```python
from build123d import *

# Parameters (mm, degrees)
SKETCH1_W                  = 84.86693599
SKETCH1_H                  = 63.5
SKETCH1_R                  = 5.08
BOSS_EXTRUDE1_DEPTH        = 3.175
F_10_32_TAPPED_HOLE1_D     = 4.0386
F_10_32_TAPPED_HOLE1_DEPTH = 11.938
F_10_32_TAPPED_HOLE1_TIP   = 1.213317848
F_10_32_TAPPED_HOLE2_D     = 4.0386
F_10_32_TAPPED_HOLE2_DEPTH = 11.938
F_10_32_TAPPED_HOLE2_TIP   = 1.213317848
SKETCH10_W                 = 84.86693599
SKETCH10_H                 = 3.175
BOSS_EXTRUDE2_DEPTH        = 22.225
F_10_32_TAPPED_HOLE3_D     = 4.0386
F_10_32_TAPPED_HOLE3_DEPTH = 11.938
F_10_32_TAPPED_HOLE3_TIP   = 1.213317848
F_10_32_TAPPED_HOLE4_D     = 4.0386
F_10_32_TAPPED_HOLE4_DEPTH = 11.938
F_10_32_TAPPED_HOLE4_TIP   = 1.213317848


with BuildPart() as part:
    # Sketch1 → Boss-Extrude1 (new body)
    with BuildSketch(Plane.XY):
        with Locations((0, -10.16)):
            Rectangle(SKETCH1_W, SKETCH1_H)
        with Locations((0, 8.89)):
            Circle(SKETCH1_R, mode=Mode.SUBTRACT)
    extrude(amount=BOSS_EXTRUDE1_DEPTH)

    # #10-32 Tapped Hole1
    with Locations(Plane.XY.offset(3.175)):
        with Locations((-19.05, 0)):
            Hole(F_10_32_TAPPED_HOLE1_D / 2, depth=F_10_32_TAPPED_HOLE1_DEPTH)
            with Locations((0, 0, -(F_10_32_TAPPED_HOLE1_DEPTH + F_10_32_TAPPED_HOLE1_TIP / 2))):  # 118° drill point
                Cone(0, F_10_32_TAPPED_HOLE1_D / 2, F_10_32_TAPPED_HOLE1_TIP, mode=Mode.SUBTRACT)

    # #10-32 Tapped Hole2
    with Locations(Plane.XY.offset(3.175)):
        with Locations((19.05, 0)):
            Hole(F_10_32_TAPPED_HOLE2_D / 2, depth=F_10_32_TAPPED_HOLE2_DEPTH)
            with Locations((0, 0, -(F_10_32_TAPPED_HOLE2_DEPTH + F_10_32_TAPPED_HOLE2_TIP / 2))):  # 118° drill point
                Cone(0, F_10_32_TAPPED_HOLE2_D / 2, F_10_32_TAPPED_HOLE2_TIP, mode=Mode.SUBTRACT)

    # Sketch10 → Boss-Extrude2 (add)
    with BuildSketch(Plane(origin=(0, 0, 0), x_dir=(-1, 0, 0), z_dir=(0, 0, -1))):
        with Locations((0, -40.3225)):
            Rectangle(SKETCH10_W, SKETCH10_H)
    extrude(amount=BOSS_EXTRUDE2_DEPTH)

    # #10-32 Tapped Hole3
    with Locations(Plane(origin=(0, -38.735, 0), x_dir=(-1, 0, 0), z_dir=(0, 1, 0))):
        with Locations((19.05, -17.78)):
            Hole(F_10_32_TAPPED_HOLE3_D / 2, depth=F_10_32_TAPPED_HOLE3_DEPTH)
            with Locations((0, 0, -(F_10_32_TAPPED_HOLE3_DEPTH + F_10_32_TAPPED_HOLE3_TIP / 2))):  # 118° drill point
                Cone(0, F_10_32_TAPPED_HOLE3_D / 2, F_10_32_TAPPED_HOLE3_TIP, mode=Mode.SUBTRACT)

    # #10-32 Tapped Hole4
    with Locations(Plane(origin=(0, -38.735, 0), x_dir=(-1, 0, 0), z_dir=(0, 1, 0))):
        with Locations((-19.05, -17.78)):
            Hole(F_10_32_TAPPED_HOLE4_D / 2, depth=F_10_32_TAPPED_HOLE4_DEPTH)
            with Locations((0, 0, -(F_10_32_TAPPED_HOLE4_DEPTH + F_10_32_TAPPED_HOLE4_TIP / 2))):  # 118° drill point
                Cone(0, F_10_32_TAPPED_HOLE4_D / 2, F_10_32_TAPPED_HOLE4_TIP, mode=Mode.SUBTRACT)


solid = part.part
```
Part model, mm, in its own coordinate system. A direction names the side the tool comes from. Coordinates: 2 decimals unless noted, no trailing zeros. Loops run counter-clockwise (first coordinate to the right, second up) from the corner with the lowest first, then second, coordinate; pieces in that order, holes last. Notation, with made-up numbers: (79, 73.5) - (101, 73.5) arc R10 cw to (101, 83.5) - close; hole circle Ø8 at (59, 1.5). An arc over 180 degrees is marked (long way). Write item = value, one per line. Start each with the question number.
Item 1: Cut at A-A, the plane x = 0. Give the cut face in (y, z) (3 decimals), and give its area (3 significant figures).
Item 2: Cut at D-D, the plane x = -19.05. Give the cut face in (y, z) (3 decimals), and give its area (3 significant figures).
Item 3: Wall check: L1, parallel to Z at x = 19.05, y = -40.15 (3 decimals); L2, parallel to Y at x = -19.05, z = 1.65; L3, parallel to Y at x = -16, z = -4 (3 decimals). Give the ranges that are in metal, low to high. Write a range as from..to.
Item 4: 3-axis set-ups, long thin cutter, end or side, ignore diameter. For faces 4 (the cylindrical face through (-0.661, 13.927, 1.565)), 5 (the flat face through (1, -38.735, -11)): which of +Z, -Z, +X, -X, +Y, -Y reach the whole face in a straight line?
Item 5: Cut at B-B, the plane z = -17.78. Give the cut face in (x, y) (3 decimals).
Item 6: Mould opens along Z. For faces 1 (the flat face through (42.433, -17, 1)), 2 (the flat face through (-1, -10, 3.175)), 3 (the cylindrical face through (-17.124, -40.345, -17.173)) say: released by +Z, released by -Z, zero draft, split by the parting line, or undercut.
Item 7: Cut at C-C, the plane y = 8.89. Give the cut face in (x, z) (3 decimals).
Item 8: Flat gauge pins, fed straight in: pin 1 Ø5 at (x, y) = (10.5, -18) entering from -Z; pin 2 Ø5.5 at (x, z) = (-19.05, -17.78) entering from +Y (3 decimals). Where does each tip first touch, or does it go through?
The answers:
q1.outline = (-41.91, -22.225) - (-38.735, -22.225) - (-38.735, 0) - (3.81, 0) - (3.81, 3.175) - (-41.91, 3.175) - close; (13.97, 0) - (21.59, 0) - (21.59, 3.175) - (13.97, 3.175) - close
q1.area = 240 mm2
q2.outline = (-41.91, -22.225) - (-38.735, -22.225) - (-38.735, -19.799) - (-41.91, -19.799) - close; (-41.91, -15.761) - (-38.735, -15.761) - (-38.735, 0) - (-2.019, 0) - (-2.019, 3.175) - (-41.91, 3.175) - close; (2.019, 0) - (21.59, 0) - (21.59, 3.175) - (2.019, 3.175) - close
q2.area = 247 mm2
q3.L1 = -22.225..-19.799, -15.761..3.175
q3.L2 = -41.91..-2.02, 2.02..21.59
q3.L3 = -41.91..-38.735
q4.face_4 = +Z, -Z
q4.face_5 = -Z, +X, -X, +Y
q5.outline = (-42.433, -41.91) - (-21.069, -41.91) - (-21.069, -38.735) - (-42.433, -38.735) - close; (-17.031, -41.91) - (17.031, -41.91) - (17.031, -38.735) - (-17.031, -38.735) - close; (21.069, -41.91) - (42.433, -41.91) - (42.433, -38.735) - (21.069, -38.735) - close
q6.face_1 = zero draft
q6.face_2 = released by +Z
q6.face_3 = undercut
q7.outline = (-42.433, 0) - (-5.08, 0) - (-5.08, 3.175) - (-42.433, 3.175) - close; (5.08, 0) - (42.433, 0) - (42.433, 3.175) - (5.08, 3.175) - close
q8.pin_1 = 0
q8.pin_2 = -38.735
